```python
from build123d import *

# Parameters (mm, degrees)
F0_W     = 2
F0_H     = 10
F1_DEPTH = 2


with BuildPart() as f1:
    # F0 (on Front) → F1 (new body)
    with BuildSketch(Plane.XZ):
        with BuildLine():
            Line((0.144111, 33.877513), (-19.580889, 33.877513))
            Line((-19.580889, 33.877513), (-21.580889, 33.877513))
            Line((-21.580889, 33.877513), (-23.753139, 33.877513))
            ThreePointArc((-23.753139, 33.877513), (-26.311046, 33.304953), (-28.380769, 31.696549))
            Line((-28.380769, 31.696549), (-62.208519, -9.293453))
            ThreePointArc((-62.208519, -9.293453), (-63.227382, -11.083423), (-63.580889, -13.112489))
            Line((-63.580889, -13.112489), (-63.580889, -20.95639))
            Line((-63.580889, -20.95639), (-53.580889, -20.95639))
            Line((-53.580889, -20.95639), (-53.580889, -22.95639))
            Line((-53.580889, -22.95639), (-39.080889, -22.95639))
            Line((-39.080889, -22.95639), (-39.080889, -20.95639))
            Line((-39.080889, -20.95639), (-21.580889, -20.95639))
            Line((-21.580889, -20.95639), (-7.330889, -20.95639))
            Line((-7.330889, -20.95639), (-7.330889, -21.122487))
            Line((-7.330889, -21.122487), (-7.330889, -22.95639))
            Line((-7.330889, -22.95639), (0.144111, -22.95639))
            Line((0.144111, -22.95639), (0.144111, 19.04361))
            ThreePointArc((0.144111, 19.04361), (-4.855889, 24.04361), (0.144111, 29.04361))
            Line((0.144111, 29.04361), (0.144111, 33.877513))
        make_face()
        with BuildLine():
            Line((-30.580889, -14.95639), (-52.737117, -14.95639))
            ThreePointArc((-52.737117, -14.95639), (-55.450837, -13.235344), (-55.050932, -10.046872))
            Line((-55.050932, -10.046872), (-32.894704, 16.800431))
            ThreePointArc((-32.894704, 16.800431), (-29.566356, 17.714159), (-27.580889, 14.890912))
            Line((-27.580889, 14.890912), (-27.580889, -11.95639))
            ThreePointArc((-27.580889, -11.95639), (-28.459568, -14.077711), (-30.580889, -14.95639))
        make_face(mode=Mode.SUBTRACT)
        with Locations((-20.580889, -10.122487)):
            Rectangle(F0_W, F0_H, mode=Mode.SUBTRACT)
        with Locations((-20.580889, 6.877513)):
            Rectangle(F0_W, F0_H, mode=Mode.SUBTRACT)
        with Locations((-20.580889, 22.877513)):
            Rectangle(F0_W, F0_H, mode=Mode.SUBTRACT)
        with BuildLine():
            Line((9.869111, 33.877513), (0.144111, 33.877513))
            Line((0.144111, 33.877513), (0.144111, 29.04361))
            ThreePointArc((0.144111, 29.04361), (3.679645, 27.579143), (5.144111, 24.04361))
            ThreePointArc((5.144111, 24.04361), (3.679645, 20.508076), (0.144111, 19.04361))
            Line((0.144111, 19.04361), (0.144111, -22.95639))
            Line((0.144111, -22.95639), (7.619111, -22.95639))
            Line((7.619111, -22.95639), (7.619111, -21.122487))
            Line((7.619111, -21.122487), (7.619111, -20.95639))
            Line((7.619111, -20.95639), (19.869111, -20.95639))
            Line((19.869111, -20.95639), (19.869111, -15.122487))
            Line((19.869111, -15.122487), (19.869111, -5.122487))
            Line((19.869111, -5.122487), (19.869111, 1.877513))
            Line((19.869111, 1.877513), (19.869111, 11.877513))
            Line((19.869111, 11.877513), (19.869111, 17.877513))
            Line((19.869111, 17.877513), (19.869111, 23.877513))
            ThreePointArc((19.869111, 23.877513), (16.940179, 30.948581), (9.869111, 33.877513))
        make_face()
    extrude(amount=F1_DEPTH)


solid = f1.part
```
Verification items for the finished model (mm, model axes). A direction names the side the tool comes from. Coordinates: 2 decimals unless noted, no trailing zeros. Loops run counter-clockwise (first coordinate to the right, second up) from the corner with the lowest first, then second, coordinate; pieces in that order, holes last. Notation, with made-up numbers: (86.25, 48) -> (106.25, 48) arc R22 cw to (106.25, 69) -> close; hole circle Ø4 at (82, 4.5). An arc over 180 degrees is marked (long way). Answer in a Markdown table with one row per item.
1) Access from +Z, -Z, +X, -X, +Y, -Y to the whole of each face (thin tool, end or side, straight path). Record for faces 1 (the face through (-59, -1, -20.956)), 2 (the face through (14, -1, -20.956)), 3 (the face through (-23, -1, -20.956)), 4 (the face through (19.869, -1, 1)), 5 (the face through (-19.581, -1, 7)).
The answers:
| item | result |
|---|---|
| face 1 | -Z, -X, +Y, -Y |
| face 2 | -Z, +X, +Y, -Y |
| face 3 | -Z, +Y, -Y |
| face 4 | +Z, -Z, +X, +Y, -Y |
| face 5 | +Y, -Y |
2) Scan lines: line 1 along Z through (x, y) = (-21, -1.5); line 2 along X through (y, z) = (-1.3, 4.5); line 3 along X through (y, z) = (-1.7, -14.5). Record each from-to range of solid material in increasing order. Write a range as from..to.
The answers:
| item | result |
|---|---|
| line 1 | z = -20.96..-15.12, -5.12..1.88, 11.88..17.88, 27.88..33.88 |
| line 2 | x = -50.83..-43.05, -27.58..-21.58, -19.58..19.87 |
| line 3 | x = -63.58..-54.33, -28.99..-21.58, -19.58..19.87 |
3) Section check B-B (z = -14). Record the cut outline in (x, y), and give its area (3 significant figures).
The answers:
| item | result |
|---|---|
| outline | (-63.58, -2) -> (-54.93, -2) -> (-54.93, 0) -> (-63.58, 0) -> close; (-28.38, -2) -> (-21.58, -2) -> (-21.58, 0) -> (-28.38, 0) -> close; (-19.58, -2) -> (19.87, -2) -> (19.87, 0) -> (-19.58, 0) -> close |
| area | 110 mm2 |
4) Section check C-C (y = -0.9). Give the number of separate pieces and of enclosed holes in the cut face, and give its area (3 significant figures).
The answers:
| item | result |
|---|---|
| separate pieces | 1 |
| enclosed holes | 5 |
| area | 3,070 mm2 |
5) Draft check along X on faces 6 (the face through (7.619, -1, -22)), 7 (the face through (-21.581, -1, 7)), 8 (the face through (-46, -1, -22.956)). Enter one of: released by +X, released by -X, zero draft, split by the parting line, or undercut.
The answers:
| item | result |
|---|---|
| face 6 | released by +X |
| face 7 | undercut |
| face 8 | zero draft |
6) Section check D-D (z = -3). Record the cut outline in (x, y), and give its area (3 significant figures).
The answers:
| item | result |
|---|---|
| outline | (-57.01, -2) -> (-49.24, -2) -> (-49.24, 0) -> (-57.01, 0) -> close; (-27.58, -2) -> (19.87, -2) -> (19.87, 0) -> (-27.58, 0) -> close |
| area | 110 mm2 |
7) Section check A-A (x = -44.5). Record the cut outline in (y, z).
The answers:
| item | result |
|---|---|
| outline | (-2, -22.96) -> (0, -22.96) -> (0, -14.96) -> (-2, -14.96) -> close; (-2, 2.74) -> (0, 2.74) -> (0, 12.16) -> (-2, 12.16) -> close |
8) Depth check by flat-ended pin: P1, Ø0.6, axis at y = -1, z = 21.5, coming from the -X side; P2, Ø0.6, axis at y = -1, z = -22, coming from the -X side; P3, Ø8, axis at x = -23, z = 20.5, coming from the +Y side; P4, Ø0.6, axis at x = -28.5, y = -0.5, coming from the -Z side. Enter the tip coordinate at first touch or a pass-through.
The answers:
| item | result |
|---|---|
| P1 | stops at x = -37.04 |
| P2 | stops at x = -53.58 |
| P3 | stops at y = 0 |
| P4 | stops at z = -20.96 |
